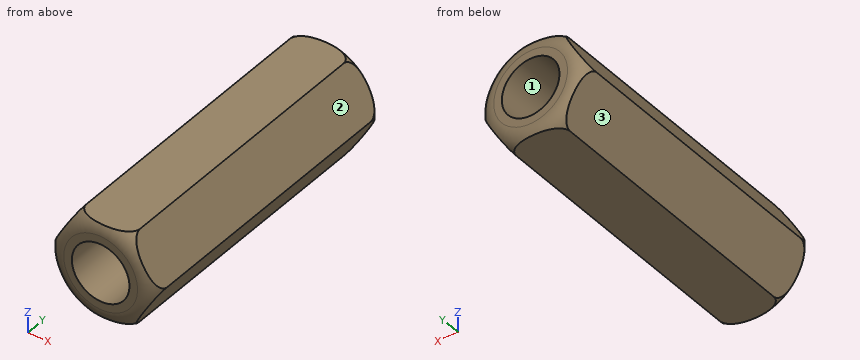
from build123d import *

# Parameters (mm, degrees)
BOSS_EXTRUDE1_DEPTH      = 18
M3_CLEARANCE_HOLE1_D     = 3.4
M3_CLEARANCE_HOLE1_DEPTH = 20
M3_CLEARANCE_HOLE1_TIP   = 1.021463052


with BuildPart() as part:
    # Sketch1 → Boss-Extrude1 (new body)
    with BuildSketch(Plane(origin=(0, 0, 0), x_dir=(1, 0, 0), z_dir=(0, 1, 0))):
        Polygon((3.175426481, 0), (1.58771324, 2.75), (-1.58771324, 2.75), (-3.175426481, 0), (-1.58771324, -2.75), (1.58771324, -2.75), align=None)
    extrude(amount=BOSS_EXTRUDE1_DEPTH)

    # M3 Clearance Hole1
    with Locations(Plane(origin=(0, 18, 0), x_dir=(-1, 0, 0), z_dir=(0, 1, 0))):
        with Locations((0, 0)):
            Hole(M3_CLEARANCE_HOLE1_D / 2, depth=M3_CLEARANCE_HOLE1_DEPTH)
            with Locations((0, 0, -(M3_CLEARANCE_HOLE1_DEPTH + M3_CLEARANCE_HOLE1_TIP / 2))):  # 118° drill point
                Cone(0, M3_CLEARANCE_HOLE1_D / 2, M3_CLEARANCE_HOLE1_TIP, mode=Mode.SUBTRACT)

    # Sketch4 → Cut-Revolve1 (revolve, cut)
    with BuildSketch(Plane.XY):
        with BuildLine():
            Line((-2.175426481, 18), (-3.175426481, 18))
            Line((-3.175426481, 18), (-3.175426481, 17))
            ThreePointArc((-3.175426481, 17), (-2.882533262, 17.707106781), (-2.175426481, 18))
        make_face()
        with BuildLine():
            Line((-3.175426481, 1), (-3.175426481, 0))
            Line((-3.175426481, 0), (-2.175426481, 0))
            ThreePointArc((-2.175426481, 0), (-2.882533262, 0.292893219), (-3.175426481, 1))
        make_face()
    revolve(axis=Axis((0, 18, 0), (0, -1, 0)), mode=Mode.SUBTRACT)


solid = part.part
CAD build for the part. Positions are in the model's coordinates, mm. Face numbers are marked on the shaded views. Coordinates: 2 decimals unless noted, no trailing zeros. Write each loop counter-clockwise with the first axis right and the second up, starting at its lowest first coordinate (ties: lowest second). Pieces come first, ordered by that corner, then holes. Notation, with made-up numbers: M 68,-4 L 116,-4 A17 cw 116,10 Z; hole C 62.5,66 d1. An arc over 180 degrees is marked long. Return JSON: item names as keys, results as strings.
Item 1: Two-plate mould, pull along Z, no slides. Class the marked faces 1, 2 and 3: +Z half, -Z half, draft (parallel to the pull), parting line (faces both ways), or undercut.
Findings below:
{"face 1": "undercut", "face 2": "+Z half", "face 3": "-Z half"}
Item 2: Slice it at A-A, the plane x = 0. Write the cut outline in (y, z).
Findings below:
{"outline": "M 0,-2.18 A1 ccw 0.18,-2.75 L 17.82,-2.75 A1 ccw 18,-2.18 L 18,-1.7 L 0,-1.7 Z; M 0,1.7 L 18,1.7 L 18,2.18 A1 ccw 17.82,2.75 L 0.18,2.75 A1 ccw 0,2.18 Z"}
Item 3: Slice it at B-B, the plane y = 14.5. Write the cut outline in (x, z), and give its area (3 significant figures).
Findings below:
{"outline": "M -3.18,0 L -1.59,-2.75 L 1.59,-2.75 L 3.18,0 L 1.59,2.75 L -1.59,2.75 Z; hole C 0,0 d3.4", "area": "17.1 mm2"}
Item 4: Drop a flat-ended pin along its axis: pin 1 Ø1.5 at (y, z) = (13.5, 1.5) entering from -X. Give the stop position or say it passes through.
Findings below:
{"pin 1": "stops at x = -2.74"}
Item 5: Probe line 1 (Z direction, x = 0, y = 7); line 2 (Z direction, x = 1.5, y = 16.25); line 3 (X direction, y = 12, z = 1.05). List the from-to ranges inside material, lowest first. Write a range as from..to.
Findings below:
{"line 1": "z = -2.75..-1.7, 1.7..2.75", "line 2": "z = -2.75..-0.8, 0.8..2.75", "line 3": "x = -2.57..-1.34, 1.34..2.57"}
